The listing builds one solid part. Answer for the finished solid, in the listing's coordinates (mm). Face numbers are marked on the shaded views. A direction names the side the tool comes from. Give positions to 0.01 mm unless a question says otherwise; leave off trailing zeros. Order: outer loops, then holes, each group sorted by start corner. A loop starts at its lowest first (then second) coordinate and runs counter-clockwise, first axis right, second up. Notation, with made-up numbers: (-8, 26) - (44, 26) arc R11 cw to (44, 43) - close; hole circle Ø10 at (-16, 85.5). An arc over 180 degrees is marked (long way). Use CSV: the item, a comma, the result in double quotes.
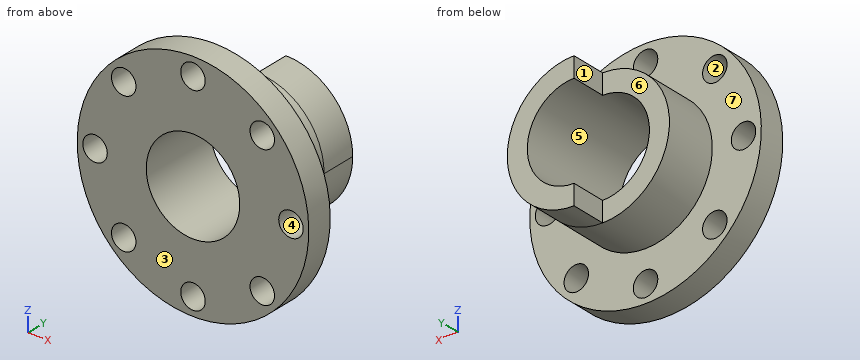
```python
from build123d import *

# Parameters (mm, degrees)
SKETCH1_R           = 13
SKETCH1_R_2         = 1.375
SKETCH1_R_3         = 5
BOSS_EXTRUDE1_DEPTH = 3
SKETCH2_R           = 7.5
SKETCH2_R_2         = 5
BOSS_EXTRUDE2_DEPTH = 10
SKETCH3_R           = 5.25
CUT_EXTRUDE1_DEPTH  = 18
CUT_EXTRUDE2_DEPTH  = 4
CUT_EXTRUDE3_START  = -10
SKETCH5_R           = 7.5
SKETCH5_R_2         = 7.45
CUT_EXTRUDE3_DEPTH  = 10
SKETCH6_R           = 7.5
SKETCH6_R_2         = 5.25
BOSS_EXTRUDE3_DEPTH = 6
BOSS_EXTRUDE4_DEPTH = 4


with BuildPart() as part:
    # Sketch1 → Boss-Extrude1 (new body)
    with BuildSketch(Plane(origin=(0, 0, 0), x_dir=(1, 0, 0), z_dir=(0, 1, 0))):
        with Locations(Location((0, 0, 0), (0, 0, 270))):
            Circle(SKETCH1_R)
        with Locations(Location((0, 11, 0), (0, 0, 270))):
            Circle(SKETCH1_R_2, mode=Mode.SUBTRACT)
        with Locations(Location((7.778174593, 7.778174593, 0), (0, 0, 270))):
            Circle(SKETCH1_R_2, mode=Mode.SUBTRACT)
        with Locations(Location((11, 0, 0), (0, 0, 270))):
            Circle(SKETCH1_R_2, mode=Mode.SUBTRACT)
        with Locations(Location((7.778174593, -7.778174593, 0), (0, 0, 270))):
            Circle(SKETCH1_R_2, mode=Mode.SUBTRACT)
        with Locations(Location((0, -11, 0), (0, 0, 270))):
            Circle(SKETCH1_R_2, mode=Mode.SUBTRACT)
        with Locations(Location((-7.778174593, -7.778174593, 0), (0, 0, 270))):
            Circle(SKETCH1_R_2, mode=Mode.SUBTRACT)
        with Locations(Location((-11, 0, 0), (0, 0, 270))):
            Circle(SKETCH1_R_2, mode=Mode.SUBTRACT)
        with Locations(Location((-7.778174593, 7.778174593, 0), (0, 0, 270))):
            Circle(SKETCH1_R_2, mode=Mode.SUBTRACT)
        with Locations(Location((0, 0, 0), (0, 0, 270))):
            Circle(SKETCH1_R_3, mode=Mode.SUBTRACT)
    extrude(amount=BOSS_EXTRUDE1_DEPTH)

    # Sketch2 → Boss-Extrude2 (add)
    with BuildSketch(Plane(origin=(0, 3, 0), x_dir=(1, 0, 0), z_dir=(0, 1, 0))):
        with Locations(Location((0, 0, 0), (0, 0, 270))):
            Circle(SKETCH2_R)
        with Locations(Location((0, 0, 0), (0, 0, 270))):
            Circle(SKETCH2_R_2, mode=Mode.SUBTRACT)
    extrude(amount=BOSS_EXTRUDE2_DEPTH)

    # Sketch3 → Cut-Extrude1 (cut)
    with BuildSketch(Plane(origin=(0, 13, 0), x_dir=(1, 0, 0), z_dir=(0, 1, 0))):
        with Locations(Location((0, 0, 0), (0, 0, 270))):
            Circle(SKETCH3_R)
    extrude(amount=-CUT_EXTRUDE1_DEPTH, mode=Mode.SUBTRACT)

    # Sketch4 → Cut-Extrude2 (cut)
    with BuildSketch(Plane(origin=(0, 13, 0), x_dir=(1, 0, 0), z_dir=(0, 1, 0))):
        with BuildLine():
            Line((0, 5.25), (0, 7.5))
            ThreePointArc((0, 7.5), (-7.5, 0), (0, -7.5))
            Line((0, -7.5), (0, -5.25))
            ThreePointArc((0, -5.25), (-5.25, 0), (0, 5.25))
        make_face()
    extrude(amount=-CUT_EXTRUDE2_DEPTH, mode=Mode.SUBTRACT)

    # Sketch5 → Cut-Extrude3 (cut)
    with BuildSketch(Plane(origin=(0, 13, 0), x_dir=(1, 0, 0), z_dir=(0, 1, 0)).offset(CUT_EXTRUDE3_START)):
        Circle(SKETCH5_R)
        with Locations(Location((0, 0, 0), (0, 0, 270))):
            Circle(SKETCH5_R_2, mode=Mode.SUBTRACT)
    extrude(amount=CUT_EXTRUDE3_DEPTH, mode=Mode.SUBTRACT)

    # Sketch6 → Boss-Extrude3 (add)
    with BuildSketch(Plane(origin=(0, 9, 0), x_dir=(1, 0, 0), z_dir=(0, 1, 0))):
        with Locations(Location((0, 0, 0), (0, 0, 270))):
            Circle(SKETCH6_R)
        with Locations(Location((0, 0, 0), (0, 0, 270))):
            Circle(SKETCH6_R_2, mode=Mode.SUBTRACT)
    extrude(amount=-BOSS_EXTRUDE3_DEPTH)

    # Sketch7 → Boss-Extrude4 (add)
    with BuildSketch(Plane(origin=(0, 9, 0), x_dir=(1, 0, 0), z_dir=(0, 1, 0))):
        with BuildLine():
            ThreePointArc((7.5, 0), (5.303300859, 5.303300859), (0, 7.5))
            Line((0, 7.5), (0, 7.45))
            ThreePointArc((0, 7.45), (5.26794552, 5.26794552), (7.45, 0))
            ThreePointArc((7.45, 0), (5.26794552, -5.26794552), (0, -7.45))
            Line((0, -7.45), (0, -7.5))
            ThreePointArc((0, -7.5), (5.303300859, -5.303300859), (7.5, 0))
        make_face()
    extrude(amount=BOSS_EXTRUDE4_DEPTH)


solid = part.part
```
Item 1: Which of the six approach directions +Z, -Z, +X, -X, +Y, -Y give full straight-line access (tool end or side, diameter ignored) to the marked faces 5, 6 and 7?
Taken from the geometry:
face 5,"+Y, -Y"
face 6,"+Z, -Z, -X, +Y"
face 7,"+Y"
Item 2: The part is cut by section D-D (z = -4.75). Give the vertices of the cut face in (x, y).
Taken from the geometry:
outline,"(-12.1, 0) - (-2.24, 0) - (-2.24, 9) - (-5.8, 9) - (-5.8, 3) - (-12.1, 3) - close; (2.24, 0) - (12.1, 0) - (12.1, 3) - (5.8, 3) - (5.8, 13) - (2.24, 13) - close"
Item 3: Find the intervals of material crossed by line 1 along Y through (x, z) = (3.5, 8.5); line 2 along X through (y, z) = (7.5, -3); line 3 along Z through (x, y) = (7, 1.25), in increasing order.
Taken from the geometry:
line 1,"0 to 3"
line 2,"-6.87 to -4.31, 4.31 to 6.87"
line 3,"-10.95 to -8.91, -6.64 to 6.64, 8.91 to 10.95"
Item 4: The part is cut by section C-C (y = 2.5). Count the separate pieces of the cut face and the enclosed holes in it, and give its area (3 significant figures).
Taken from the geometry:
separate pieces,"1"
enclosed holes,"9"
area,"397 mm^2"
Item 5: Each of these flat-tipped pins is pushed along its axis until it touches: pin 1 (2 mm diameter, centred on y = 9.5, z = -6, fed in from +X); pin 2 (2 mm diameter, centred on y = 3, z = 2.5, fed in from +X); pin 3 (2 mm diameter, centred on x = 11, z = 0, fed in from +Y); pin 4 (3 mm diameter, centred on x = -7.78, z = 7.78, fed in from +Y). Where does it stop, or does it pass through?
Taken from the geometry:
pin 1,"x = 5.59"
pin 2,"x = 12.91"
pin 3,"through"
pin 4,"y = 3"
Item 6: The part is cut by section B-B (x = 4.5). Give the vertices of the cut face in (y, z).
Taken from the geometry:
outline,"(0, -12.2) - (3, -12.2) - (3, -6) - (13, -6) - (13, -2.7) - (0, -2.7) - close; (0, 2.7) - (13, 2.7) - (13, 6) - (3, 6) - (3, 12.2) - (0, 12.2) - close"
Item 7: The part is cut by section A-A (z = 8.25). Give the vertices of the cut face in (x, y), and give its area (3 significant figures).
Taken from the geometry:
outline,"(-10.05, 0) - (-9.07, 0) - (-9.07, 3) - (-10.05, 3) - close; (-6.49, 0) - (6.49, 0) - (6.49, 3) - (-6.49, 3) - close; (9.07, 0) - (10.05, 0) - (10.05, 3) - (9.07, 3) - close"
area,"44.8 mm^2"
Item 8: The mould has two halves that part along X. Classify the marked faces 1, 2, 3 and 4: +X half, -X half, draft (parallel to the pull), parting line (faces both ways), or undercut.
Taken from the geometry:
face 1,"-X half"
face 2,"undercut"
face 3,"draft"
face 4,"undercut"
